Verification items for the finished model (mm, model axes). Coordinates: 2 decimals unless noted, no trailing zeros. Order: outer loops, then holes, each group sorted by start corner. A loop starts at its lowest first (then second) coordinate and runs counter-clockwise, first axis right, second up. Notation, with made-up numbers: (62.5, 66.25) -> (118.5, 66.25) arc R11 ccw to (118.5, 87.25) -> close; hole circle Ø9 at (52, -20.75). An arc over 180 degrees is marked (long way). Write item = value, one per line. Start each with the question number.
1. Thickness scan on line 1 along X through (y, z) = (-15, 13); line 2 along Z through (x, y) = (-3, -8). Record the ranges inside material, lowest first. Write a range as from..to.
2. Cross-section at B-B on y = 3. Record the cut outline in (x, z), plus the area to 3 significant figures.
3. Go/stop test with flat-tipped pins: P1, Ø12, axis at x = 9, y = -7, coming from the -Z side; P2, Ø5, axis at x = -0.5, y = 2, coming from the -Z side. Record where each tip stops, or that it passes through.
4. Cross-section at A-A on z = 24. Record the cut outline in (x, y).
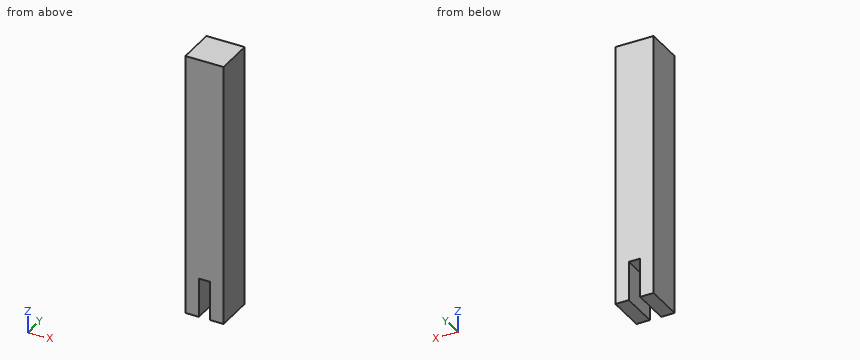
from build123d import *

# Parameters (mm, degrees)
SKETCH_W     = 34
SKETCH_H     = 34
PAD_DEPTH    = 235
SKETCH001_W  = 10
SKETCH001_H  = 34
POCKET_DEPTH = 35


with BuildPart() as part:
    # Sketch → Pad (new body)
    with BuildSketch(Plane.XY):
        Rectangle(SKETCH_W, SKETCH_H)
    extrude(amount=PAD_DEPTH)

    # Sketch001 → Pocket (cut)
    with BuildSketch(Plane.XY):
        Rectangle(SKETCH001_W, SKETCH001_H)
    extrude(amount=POCKET_DEPTH, mode=Mode.SUBTRACT)


solid = part.part
Worked out:
q1.line_1 = -17..-5, 5..17
q1.line_2 = 35..235
q2.outline = (-17, 0) -> (-5, 0) -> (-5, 35) -> (5, 35) -> (5, 0) -> (17, 0) -> (17, 235) -> (-17, 235) -> close
q2.area = 7,640 mm²
q3.P1 = 0
q3.P2 = 35
q4.outline = (-17, -17) -> (-5, -17) -> (-5, 17) -> (-17, 17) -> close; (5, -17) -> (17, -17) -> (17, 17) -> (5, 17) -> close
